```python
from build123d import *

# Parameters (mm, degrees)
SKETCH_1_R          = 5
EXTRUDE_1_DEPTH     = 15
CUT_EXTRUDE_START   = -4
SKETCH_2_R          = 5
SKETCH_2_R_2        = 3
CUT_EXTRUDE_1_DEPTH = 4
SKETCH_3_R          = 5
CUT_EXTRUDE_2_DEPTH = 25
SKETCH_4_R          = 1.6
CUT_EXTRUDE_3_DEPTH = 17.583123952
SKETCH_5_R          = 5
SKETCH_5_R_2        = 3
CUT_EXTRUDE_4_DEPTH = 2.1
SKETCH_6_OUTSIDE_W  = 16.124
SKETCH_6_OUTSIDE_H  = 16.124
SKETCH_6_OUTSIDE_R  = 3
CUT_EXTRUDE_5_DEPTH = 3
CUT_EXTRUDE_START_2 = -1.8
SKETCH_7_R          = 3
CUT_EXTRUDE_6_DEPTH = 1.8


with BuildPart() as part:
    # 草图1 → 凸台-拉伸1 (new body)
    with BuildSketch(Plane.XY):
        Circle(SKETCH_1_R)
    extrude(amount=EXTRUDE_1_DEPTH)

    # 草图2 → 切除-拉伸1 (cut)
    with BuildSketch(Plane.XY.offset(13).offset(CUT_EXTRUDE_START)):
        Circle(SKETCH_2_R)
        Circle(SKETCH_2_R_2, mode=Mode.SUBTRACT)
    extrude(amount=CUT_EXTRUDE_1_DEPTH, mode=Mode.SUBTRACT)

    # 草图3 → 切除-拉伸2 (cut, symmetric)
    with BuildSketch(Plane(origin=(0, 0, 0), x_dir=(1, 0, 0), z_dir=(0, 1, 0))):
        with Locations((0, 2)):
            Circle(SKETCH_3_R)
    extrude(amount=CUT_EXTRUDE_2_DEPTH, both=True, mode=Mode.SUBTRACT)

    # 草图4 → 切除-拉伸3 (cut, through all)
    with BuildSketch(Plane.XY.offset(15)):
        Circle(SKETCH_4_R)
    extrude(amount=-CUT_EXTRUDE_3_DEPTH, mode=Mode.SUBTRACT)

    # 草图5 → 切除-拉伸4 (cut, symmetric)
    with BuildSketch(Plane.XY.offset(11)):
        with Locations(Location((0, 0, 0), (0, 0, 203.578178478))):
            Circle(SKETCH_5_R)
        Circle(SKETCH_5_R_2, mode=Mode.SUBTRACT)
    extrude(amount=CUT_EXTRUDE_4_DEPTH, both=True, mode=Mode.SUBTRACT)

    # 草图6 outside → 切除-拉伸5 (cut)
    with BuildSketch(Plane.XY.offset(15)):
        Rectangle(SKETCH_6_OUTSIDE_W, SKETCH_6_OUTSIDE_H)
        Circle(SKETCH_6_OUTSIDE_R, mode=Mode.SUBTRACT)
    extrude(amount=-CUT_EXTRUDE_5_DEPTH, mode=Mode.SUBTRACT)

    # 草图7 → 切除-拉伸6 (cut)
    with BuildSketch(Plane.XY.offset(15).offset(CUT_EXTRUDE_START_2)):
        Circle(SKETCH_7_R)
    extrude(amount=CUT_EXTRUDE_6_DEPTH, mode=Mode.SUBTRACT)


solid = part.part
```
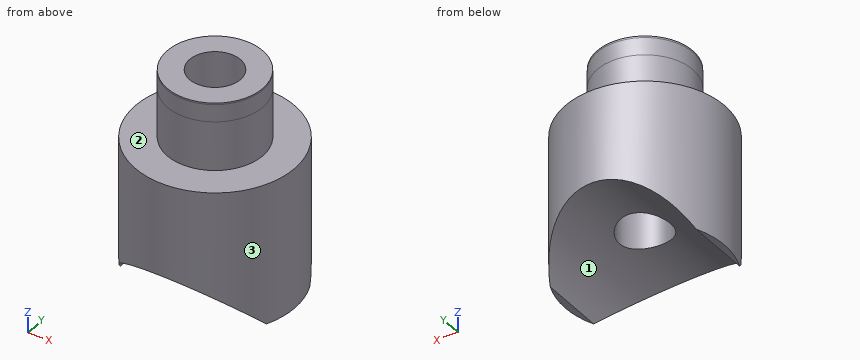
Build history of the part. All positions in model axes, mm. Face numbers are marked on the shaded views. Give positions to 0.01 mm unless a question says otherwise; leave off trailing zeros. Loops run counter-clockwise (first coordinate to the right, second up) from the corner with the lowest first, then second, coordinate; pieces in that order, holes last.
1) Drop flat-ended pins along their axis: P1, Ø5, axis at x = 3.5, y = 3.5, coming from the +Z side; P2, Ø1, axis at y = -3.5, z = 5, coming from the +X side; P3, Ø4, axis at x = 2, z = 12, coming from the +Y side; P4, Ø3.5, axis at x = 0, y = 0, coming from the -Z side. Give the stop position or say it passes through.
Values follow:
P1: stops at z = 13.2
P2: stops at x = 4
P3: stops at y = 3
P4: stops at z = 2.68
2) Two-plate mould, pull along X, no slides. Class the marked faces 1, 2 and 3: released by +X, released by -X, zero draft, split by the parting line, or undercut.
Values follow:
face 1: undercut
face 2: zero draft
face 3: split by the parting line
3) Band-saw the part on C-C on z = 11. List the corners of the cut face in (x, y).
Values follow:
outline: circle Ø6 at (0, 0); hole circle Ø3.2 at (0, 0)
4) Band-saw the part on D-D on x = -1. List the corners of the cut face in (y, z).
Values follow:
outline: (-4.9, 2.9) - (-1.25, 2.9) - (-1.25, 13.2) - (-2.83, 13.2) - (-2.83, 8.9) - (-4.9, 8.9) - close; (1.25, 2.9) - (4.9, 2.9) - (4.9, 8.9) - (2.83, 8.9) - (2.83, 13.2) - (1.25, 13.2) - close
5) Probe line 1 along Y through (x, z) = (0, 8.5); line 2 along X through (y, z) = (2, 7.25). List the from-to ranges inside material, lowest first.
Values follow:
line 1: y = -5 to -1.6, 1.6 to 5
line 2: x = -4.58 to 4.58
6) Band-saw the part on B-B on y = 0. List the corners of the cut face in (x, z), then the cut area to 3 significant figures.
Values follow:
outline: (-5, 0) - (-4.58, 0) arc R5 cw to (-1.6, 2.74) - (-1.6, 13.2) - (-3, 13.2) - (-3, 8.9) - (-5, 8.9) - close; (1.6, 2.74) arc R5 cw to (4.58, 0) - (5, 0) - (5, 8.9) - (3, 8.9) - (3, 13.2) - (1.6, 13.2) - close
area: 62.1 mm2
7) Band-saw the part on A-A on x = 0. List the corners of the cut face in (y, z).
Values follow:
outline: (-5, 3) - (-1.6, 3) - (-1.6, 13.2) - (-3, 13.2) - (-3, 8.9) - (-5, 8.9) - close; (1.6, 3) - (5, 3) - (5, 8.9) - (3, 8.9) - (3, 13.2) - (1.6, 13.2) - close
